from build123d import *

# Parameters (mm, degrees)
SKETCH_1_W        = 8
SKETCH_1_H        = 8
SKETCH_1_R        = 1.25
EXTRUDE_349_DEPTH = 40
CHAMFER_1_SIZE    = 1


with BuildPart() as part:
    # Эскиз1 → Extrude 349 (new body)
    with BuildSketch(Plane(origin=(0, 0, 0), x_dir=(1, 0, 0), z_dir=(0, 1, 0))):
        Rectangle(SKETCH_1_W, SKETCH_1_H)
        with Locations(Location((0, 0, 0), (0, 0, 270))):
            Circle(SKETCH_1_R, mode=Mode.SUBTRACT)
    extrude(amount=EXTRUDE_349_DEPTH)

    # Фаска1
    chamfer_1_edges = [part.edges().sort_by_distance(p)[0] for p in [
        (4, 20, 4),
        (-4, 20, 4),
        (-4, 20, -4),
        (4, 20, -4),
    ]]
    chamfer(chamfer_1_edges, length=CHAMFER_1_SIZE)


solid = part.part
Geometry: final body of the model. Coordinates: model frame, mm. Give positions to 0.01 mm unless a question says otherwise; leave off trailing zeros. Write each loop counter-clockwise with the first axis right and the second up, starting at its lowest first coordinate (ties: lowest second). Pieces come first, ordered by that corner, then holes. Notation, with made-up numbers: (-19.5, 88) - (36.5, 88) arc R37 cw to (36.5, 126) - close; hole circle Ø3 at (84.5, 11). An arc over 180 degrees is marked (long way). Return JSON: item names as keys, results as strings. Group by question number.
1) Section C-C on y = 14. Return the cut outline in (x, z), plus the area to 3 significant figures.
2) Section B-B on z = 0. Return the cut outline in (x, y).
3) Mould query, pull axis Z, two halves, no side actions, for faces 1 (the cylindrical face through (-1.22, 19.72, -0.27)), 2 (the flat face through (0, 20, 4)), 3 (the flat face through (1, 40, -1)). Classes: released by +Z, released by -Z, zero draft, split by the parting line, or undercut.
4) Line query: line 1 (X direction, y = 24, z = 0); line 2 (Z direction, x = 0.75, y = 17.5); line 3 (X direction, y = 4, z = -0.5). Output: solid intervals per line, ascending.
5) Section A-A on x = 0. Return the cut outline in (y, z).
Filled in:
{
 "1": {"outline": "(-4, -3) - (-3, -4) - (3, -4) - (4, -3) - (4, 3) - (3, 4) - (-3, 4) - (-4, 3) - close; hole circle Ø2.5 at (0, 0)", "area": "57.1 mm^2"},
 "2": {"outline": "(-4, 0) - (-1.25, 0) - (-1.25, 40) - (-4, 40) - close; (1.25, 0) - (4, 0) - (4, 40) - (1.25, 40) - close"},
 "3": {"face 1": "undercut", "face 2": "released by +Z", "face 3": "zero draft"},
 "4": {"line 1": "x = -4 to -1.25, 1.25 to 4", "line 2": "z = -4 to -1, 1 to 4", "line 3": "x = -4 to -1.15, 1.15 to 4"},
 "5": {"outline": "(0, -4) - (40, -4) - (40, -1.25) - (0, -1.25) - close; (0, 1.25) - (40, 1.25) - (40, 4) - (0, 4) - close"}
}
